Verification items for the finished model (mm, model axes). A direction names the side the tool comes from. Coordinates: 2 decimals unless noted, no trailing zeros. Write each loop counter-clockwise with the first axis right and the second up, starting at its lowest first coordinate (ties: lowest second). Pieces come first, ordered by that corner, then holes. Notation, with made-up numbers: M 61.25,74 L 92.25,74 A5 ccw 92.25,81 Z; hole C -29,63 d4. An arc over 180 degrees is marked long. Answer in a Markdown table with one row per item.
from build123d import *

# Parameters (mm, degrees)
SKETCH1_R           = 2.5
SKETCH1_R_2         = 1.65
BOSS_EXTRUDE1_DEPTH = 2


with BuildPart() as part:
    # Sketch1 → Boss-Extrude1 (new, symmetric)
    with BuildSketch(Plane.XY):
        with BuildLine():
            Line((0, -40), (0, 40))
            Line((0, 40), (-23.37, 40))
            ThreePointArc((-23.37, 40), (-27.223373178, 38.84392977), (-29.803954922, 35.757575758))
            Line((-29.803954922, 35.757575758), (-41.752728349, 7.878787879))
            ThreePointArc((-41.752728349, 7.878787879), (-43.37, 0), (-41.752728349, -7.878787879))
            Line((-41.752728349, -7.878787879), (-29.803954922, -35.757575758))
            ThreePointArc((-29.803954922, -35.757575758), (-27.223373178, -38.84392977), (-23.37, -40))
            Line((-23.37, -40), (0, -40))
        make_face()
        with Locations((-16.37, 30)):
            Circle(SKETCH1_R, mode=Mode.SUBTRACT)
        with Locations((-16.37, -30)):
            Circle(SKETCH1_R, mode=Mode.SUBTRACT)
        with Locations((-23.37, -15.5)):
            Circle(SKETCH1_R_2, mode=Mode.SUBTRACT)
        with Locations((-36.793393759, -7.75)):
            Circle(SKETCH1_R_2, mode=Mode.SUBTRACT)
        with Locations((-36.793393759, 7.75)):
            Circle(SKETCH1_R_2, mode=Mode.SUBTRACT)
        with Locations((-23.37, 15.5)):
            Circle(SKETCH1_R_2, mode=Mode.SUBTRACT)
        with Locations((-9.946606241, 7.75)):
            Circle(SKETCH1_R_2, mode=Mode.SUBTRACT)
        with Locations((-9.946606241, -7.75)):
            Circle(SKETCH1_R_2, mode=Mode.SUBTRACT)
        with BuildLine():
            Line((-30.37, 6.6), (-16.37, 6.6))
            ThreePointArc((-16.37, 6.6), (-9.77, 0), (-16.37, -6.6))
            Line((-16.37, -6.6), (-30.37, -6.6))
            ThreePointArc((-30.37, -6.6), (-36.97, 0), (-30.37, 6.6))
        make_face(mode=Mode.SUBTRACT)
    extrude(amount=BOSS_EXTRUDE1_DEPTH, both=True)


solid = part.part
1) Thickness scan on L1, parallel to Y at x = -15.5, z = -1.2; L2, parallel to Y at x = -17.5, z = -1.8; L3, parallel to Y at x = -19, z = 0. Record the ranges inside material, lowest first. Write a range as [from, to].
Response values:
| item | result |
|---|---|
| L1 | y = [-40, -32.34], [-27.66, -6.54], [6.54, 27.66], [32.34, 40] |
| L2 | y = [-40, -32.23], [-27.77, -6.6], [6.6, 27.77], [32.23, 40] |
| L3 | y = [-40, -6.6], [6.6, 40] |
2) Sectioned sample at D-D (x = -41). Record the cut outline in (y, z), then the cut area to 3 significant figures.
Response values:
| item | result |
|---|---|
| outline | M -9.64,-2 L 9.64,-2 L 9.64,2 L -9.64,2 Z |
| area | 77.1 mm² |
3) Sectioned sample at C-C (y = -30). Record the cut outline in (x, z).
Response values:
| item | result |
|---|---|
| outline | M -32.27,-2 L -18.87,-2 L -18.87,2 L -32.27,2 Z; M -13.87,-2 L 0,-2 L 0,2 L -13.87,2 Z |
4) Release check for a two-part mould opening along Y. For faces 1 (the face through (-35.7, 22, 0)), 2 (the face through (-43.37, 0.11, 0.03)), 3 (the face through (-27.271, -38.812, 0.028)), 4 (the face through (-11.16, 8.87, -0.03)) record: +Y half, -Y half, draft (parallel to the pull), parting line (faces both ways), or undercut.
Response values:
| item | result |
|---|---|
| face 1 | +Y half |
| face 2 | parting line |
| face 3 | -Y half |
| face 4 | undercut |
5) Sectioned sample at A-A (y = 0). Record the cut outline in (x, z), then the cut area to 3 significant figures.
Response values:
| item | result |
|---|---|
| outline | M -43.37,-2 L -36.97,-2 L -36.97,2 L -43.37,2 Z; M -9.77,-2 L 0,-2 L 0,2 L -9.77,2 Z |
| area | 64.7 mm² |
6) Tool access check on faces 5 (the face through (-36.97, -0.15, 0.03)), 6 (the face through (-35.862, -21.623, 0.028)). Record the directions out of +Z, -Z, +X, -X, +Y, -Y that give a thin tool (end or side, any length) a straight path to the whole face; none if there is none.
Response values:
| item | result |
|---|---|
| face 5 | +Z, -Z |
| face 6 | +Z, -Z, -X, -Y |
7) Sectioned sample at B-B (z = 1.2). Give the number of separate pieces and of enclosed holes in the cut face, then the cut area to 3 significant figures.
Response values:
| item | result |
|---|---|
| separate pieces | 1 |
| enclosed holes | 9 |
| area | 2,500 mm² |
